The model under review builds one solid part; all positions refer to its coordinate system, in mm. A direction names the side the tool comes from. Round coordinates to 2 decimals unless told otherwise and drop trailing zeros. Write each loop counter-clockwise with the first axis right and the second up, starting at its lowest first coordinate (ties: lowest second). Pieces come first, ordered by that corner, then holes. Notation, with made-up numbers: (37.5, 63.5) -> (64.5, 63.5) arc R22 cw to (64.5, 81.5) -> close; hole circle Ø10 at (73.5, 88). An arc over 180 degrees is marked (long way). Use CSV: the item, a comma, the result in double quotes. Start each with the question number.
1) Take a section at A-A, the plane z = -36. Give the boundary of the cut face in (x, y), then the cut area to 3 significant figures.
2) Take a section at D-D, the plane y = 1.5. State how many separate pieces and enclosed holes the cut face has, then the cut area to 3 significant figures.
3) Take a section at C-C, the plane x = 91.5. Give the boundary of the cut face in (y, z).
4) Wall thickness on probe 1 along X at (y, z) = (1.25, -65); probe 2 along Z at (x, y) = (81.5, 6); probe 3 along X at (y, z) = (6.25, -64.5): over which ranges is each line inside the solid? List them lowest first. Write a range as [from, to].
5) Mouldability with a two-part tool opening along X and no side actions: class faces 1 (the face through (80.84, 3.94, -90.28)), 2 (the face through (29.5, 3.94, -65.93)), 3 (the face through (59.905, 4, -115)) as released by +X, released by -X, zero draft, split by the parting line, or undercut.
6) For pin 1 Ø4 at (y, z) = (2, -116) entering from +X; pin 2 Ø4 at (x, y) = (62.5, 2.5) entering from +Z; pin 3 Ø1 at (x, y) = (83.5, 5.5) entering from -Z, all flat-tipped, find the tip position at first contact; note any pin that passes through.
7) Machinability: for faces 4 (the face through (68.405, 4, -92)), 5 (the face through (52, 4, -110.142)), 6 (the face through (64, 4, -43.392)), which of the approach directions +Z, -Z, +X, -X, +Y, -Y give a long, thin tool a straight path to every point of the face, cutting with its end or side? Answer none if there is none.
8) Take a section at B-B, the plane z = -59. Give the boundary of the cut face in (x, y).
from build123d import *

# Parameters (mm, degrees)
SKETCH1_R      = 6.125
SKETCH1_R_2    = 4.25
SKETCH1_R_3    = 1.75
EXTRUDE1_DEPTH = 8
SKETCH3_W      = 8.5
SKETCH3_H      = 15
SKETCH3_W_2    = 15.5
SKETCH3_H_2    = 8.5
SKETCH3_H_3    = 15.5
EXTRUDE2_DEPTH = 10


with BuildPart() as part:
    # Sketch1 → Extrude1 (new body)
    with BuildSketch(Plane(origin=(0, 0, 0), x_dir=(1, 0, 0), z_dir=(0, 1, 0))):
        with BuildLine():
            Line((135.905429433, 28.391828159), (135.905429433, 74.65063841))
            ThreePointArc((135.905429433, 74.65063841), (134.908812883, 77.646121835), (132.316261053, 79.447465917))
            Line((132.316261053, 79.447465917), (67.905429433, 98.391828159))
            Line((67.905429433, 98.391828159), (59.905429433, 100.744769335))
            Line((59.905429433, 100.744769335), (59.905429433, 109.891828159))
            Line((59.905429433, 109.891828159), (59.905429433, 120.391828159))
            ThreePointArc((59.905429433, 120.391828159), (59.612536214, 121.09893494), (58.905429433, 121.391828159))
            Line((58.905429433, 121.391828159), (45.210651279, 121.391828159))
            ThreePointArc((45.210651279, 121.391828159), (44.908922851, 121.368937148), (44.614101292, 121.300788115))
            Line((44.614101292, 121.300788115), (6.308879447, 109.330406288))
            ThreePointArc((6.308879447, 109.330406288), (5.294048042, 108.606119288), (4.905429433, 107.421446332))
            Line((4.905429433, 107.421446332), (4.905429433, 101.524813665))
            ThreePointArc((4.905429433, 101.524813665), (4.998649565, 100.921331655), (5.269619969, 100.374106318))
            Line((5.269619969, 100.374106318), (54.411845802, 30.515059791))
            ThreePointArc((54.411845802, 30.515059791), (56.197442578, 28.954270168), (58.501369461, 28.391828159))
            Line((58.501369461, 28.391828159), (59.905429433, 28.391828159))
            Line((59.905429433, 28.391828159), (67.905429433, 28.391828159))
            Line((67.905429433, 28.391828159), (135.905429433, 28.391828159))
        make_face()
        with Locations(Location((127.405429433, 59.891828159, 0), (0, 0, 270))):
            Circle(SKETCH1_R, mode=Mode.SUBTRACT)
        with Locations(Location((127.405429433, 36.891828159, 0), (0, 0, 270))):
            Circle(SKETCH1_R_2, mode=Mode.SUBTRACT)
        with Locations(Location((116.798827433, 47.498429876, 0), (0, 0, 270))):
            Circle(SKETCH1_R_3, mode=Mode.SUBTRACT)
        with Locations(Location((81.905429433, 78.891828159, 0), (0, 0, 270))):
            Circle(SKETCH1_R, mode=Mode.SUBTRACT)
        with Locations(Location((81.905429433, 88.891828159, 0), (0, 0, 270))):
            Circle(SKETCH1_R_3, mode=Mode.SUBTRACT)
        with Locations(Location((81.905429433, 68.891828159, 0), (0, 0, 270))):
            Circle(SKETCH1_R_3, mode=Mode.SUBTRACT)
        with Locations(Location((38.905429433, 83.391828159, 0), (0, 0, 270))):
            Circle(SKETCH1_R, mode=Mode.SUBTRACT)
        with Locations(Location((38.905429433, 93.391828159, 0), (0, 0, 270))):
            Circle(SKETCH1_R_3, mode=Mode.SUBTRACT)
        with Locations(Location((38.905429433, 73.391828159, 0), (0, 0, 270))):
            Circle(SKETCH1_R_3, mode=Mode.SUBTRACT)
        with Locations(Location((35.405429433, 105.891828159, 0), (0, 0, 270))):
            Circle(SKETCH1_R_3, mode=Mode.SUBTRACT)
        with Locations(Location((63.905429433, 65.891828159, 0), (0, 0, 270))):
            Circle(SKETCH1_R_3, mode=Mode.SUBTRACT)
    extrude(amount=EXTRUDE1_DEPTH)

    # Sketch3 → Extrude2 (cut)
    with BuildSketch(Plane(origin=(0, 8, 0), x_dir=(1, 0, 0), z_dir=(0, 1, 0))):
        with Locations((63.905429433, 35.891828159)):
            Rectangle(SKETCH3_W, SKETCH3_H)
        with Locations((52.155429433, 105.891828159)):
            Rectangle(SKETCH3_W_2, SKETCH3_H_2)
        with Locations((64.155429433, 93.891828159)):
            Rectangle(SKETCH3_W, SKETCH3_H_3)
    extrude(amount=-EXTRUDE2_DEPTH, mode=Mode.SUBTRACT)


solid = part.part
Values found:
1,outline,"(50.55, 0) -> (59.66, 0) -> (59.66, 8) -> (50.55, 8) -> close; (68.16, 0) -> (123.25, 0) -> (123.25, 8) -> (68.16, 8) -> close; (131.56, 0) -> (135.91, 0) -> (135.91, 8) -> (131.56, 8) -> close"
1,area,"548 mm²"
2,separate pieces,"1"
2,enclosed holes,"11"
2,area,"6,810 mm²"
3,outline,"(0, -91.45) -> (8, -91.45) -> (8, -28.39) -> (0, -28.39) -> close"
4,probe 1,"[30.15, 62.4], [65.41, 124.03], [130.79, 135.91]"
4,probe 2,"[-94.39, -90.59], [-87.19, -85], [-72.78, -70.59], [-67.19, -28.39]"
4,probe 3,"[30.51, 62.84], [64.97, 123.37], [131.44, 135.91]"
5,face 1,"undercut"
5,face 2,"released by -X"
5,face 3,"released by +X"
6,pin 1,"x = 59.91"
6,pin 2,"z = -43.39"
6,pin 3,"z = -93.95"
7,face 4,"-Z, +Y, -Y"
7,face 5,"+X, +Y, -Y"
7,face 6,"+Z, +Y, -Y"
8,outline,"(34.37, 0) -> (121.35, 0) -> (121.35, 8) -> (34.37, 8) -> close; (133.47, 0) -> (135.91, 0) -> (135.91, 8) -> (133.47, 8) -> close"
